from build123d import *

# Parameters (mm, degrees)
F1_DEPTH = 20
F2_R     = 10
F3_R     = 2
F4_DEPTH = 30


with BuildPart() as f1:
    # F0 (on Top) → F1 (new body)
    with BuildSketch(Plane.XY):
        with BuildLine():
            ThreePointArc((-11, 0), (0, 11), (11, 0))
            Line((11, 0), (15, 0))
            ThreePointArc((15, 0), (0, 15), (-15, 0))
            Line((-15, 0), (-11, 0))
        make_face()
        with BuildLine():
            Line((15, 0), (11, 0))
            Line((11, 0), (11, -10.1980390272))
            ThreePointArc((11, -10.1980390272), (13.9642400438, -5.4772255751), (15, 0))
        make_face()
        with BuildLine():
            Line((-11, -10.1980390272), (-11, 0))
            Line((-11, 0), (-15, 0))
            ThreePointArc((-15, 0), (-13.9642400438, -5.4772255751), (-11, -10.1980390272))
        make_face()
        with BuildLine():
            Line((11, -10.1980390272), (11, 0))
            ThreePointArc((11, 0), (0, -11), (-11, 0))
            Line((-11, 0), (-11, -10.1980390272))
            ThreePointArc((-11, -10.1980390272), (0, -15), (11, -10.1980390272))
        make_face()
        with BuildLine():
            ThreePointArc((-11, -10.1980390272), (-13.9642400438, -5.4772255751), (-15, 0))
            Line((-15, 0), (-15, -35))
            Line((-15, -35), (-11, -35))
            Line((-11, -35), (-11, -10.1980390272))
        make_face()
        with BuildLine():
            Line((15, -35), (15, 0))
            ThreePointArc((15, 0), (13.9642400438, -5.4772255751), (11, -10.1980390272))
            Line((11, -10.1980390272), (11, -35))
            Line((11, -35), (15, -35))
        make_face()
    extrude(amount=F1_DEPTH)

    # F2
    f2_edges = [f1.edges().sort_by_distance(p)[0] for p in [
        (-13, -35, 20),
        (13, -35, 20),
    ]]
    fillet(f2_edges, radius=F2_R)

    # F3 (on face) → F4 (cut)
    with BuildSketch(Plane.YZ.offset(15)):
        with Locations((-25, 10)):
            Circle(F3_R)
        with BuildLine():
            ThreePointArc((0, 8), (1.4142135624, 8.5857864376), (2, 10))
            ThreePointArc((2, 10), (1.4142135624, 11.4142135624), (0, 12))
            Line((0, 12), (0, 8))
        make_face()
        with BuildLine():
            Line((0, 8), (0, 12))
            ThreePointArc((0, 12), (-2, 10), (0, 8))
        make_face()
    extrude(amount=-F4_DEPTH, mode=Mode.SUBTRACT)


solid = f1.part
Verification items for the finished model (mm, model axes). A direction names the side the tool comes from. Coordinates: 2 decimals unless noted, no trailing zeros. Write each loop counter-clockwise with the first axis right and the second up, starting at its lowest first coordinate (ties: lowest second). Pieces come first, ordered by that corner, then holes. Notation, with made-up numbers: M 78.5,-17 L 127.5,-17 A12 ccw 127.5,1 Z; hole C 12,44.25 d11. An arc over 180 degrees is marked long. Use a Markdown table: item, result.
Q1. Sectioned sample at B-B, the plane y = -21.5. Record the boundary of the cut face in (x, z).
Reply:
| item | result |
|---|---|
| outline | M -15,0 L -11,0 L -11,20 L -15,20 Z; M 11,0 L 15,0 L 15,20 L 11,20 Z |
Q2. Set-up check for faces 4 (the face through (-11, -22.8, 9.9)), 5 (the face through (10.161, 4.213, 9.86)): record each of +Z, -Z, +X, -X, +Y, -Y from which the full face is reachable in a straight line by a thin tool's end or side.
Reply:
| item | result |
|---|---|
| face 4 | +Z, -Z, -Y |
| face 5 | +Z, -Z |
Q3. Sectioned sample at D-D, the plane y = -1.5. Record the boundary of the cut face in (x, z), plus the area to 3 significant figures.
Reply:
| item | result |
|---|---|
| outline | M -15,0 L -10.9,0 L -10.9,8.68 L -15,8.68 Z; M -15,11.32 L -10.9,11.32 L -10.9,20 L -15,20 Z; M 10.9,0 L 15,0 L 15,8.68 L 10.9,8.68 Z; M 10.9,11.32 L 15,11.32 L 15,20 L 10.9,20 Z |
| area | 142 mm² |
Q4. Sectioned sample at C-C, the plane x = -7. Record the boundary of the cut face in (y, z).
Reply:
| item | result |
|---|---|
| outline | M -13.27,0 L -8.49,0 L -8.49,20 L -13.27,20 Z; M 8.49,0 L 13.27,0 L 13.27,20 L 8.49,20 Z |
Q5. Go/stop test with flat-tipped pins: P1, Ø1, axis at x = 7, z = 5, coming from the +Y side; P2, Ø8, axis at x = -5, z = 15, coming from the -Y side; P3, Ø10, axis at x = 12, z = 17.5, coming from the -Y side; P4, Ø12, axis at x = 0.5, y = -11, coming from the -Z side. Record where each tip stops, or that it passes through.
Reply:
| item | result |
|---|---|
| P1 | stops at y = 13.52 |
| P2 | stops at y = -14.97 |
| P3 | stops at y = -34.68 |
| P4 | stops at z = 0 |
Q6. Thickness scan on line 1 (X direction, y = -21, z = 8.5); line 2 (Z direction, x = -12.25, y = -25). Record the ranges inside material, lowest first.
Reply:
| item | result |
|---|---|
| line 1 | x = -15 to -11, 11 to 15 |
| line 2 | z = 0 to 8, 12 to 20 |
Q7. Sectioned sample at A-A, the plane z = 16. Record the boundary of the cut face in (x, y).
Reply:
| item | result |
|---|---|
| outline | M -15,-33 L -11,-33 L -11,-10.2 A15 ccw 11,-10.2 L 11,-33 L 15,-33 L 15,0 A15 ccw -15,0 Z; hole C 0,0 d22 |
Q8. Draft check along Y on faces 1 (the face through (-13, -35, 5)), 2 (the face through (11, -22, 10)), 3 (the face through (-12.972, -26.474, 11.352)). Enter one of: +Y half, -Y half, draft (parallel to the pull), parting line (faces both ways), or undercut.
Reply:
| item | result |
|---|---|
| face 1 | -Y half |
| face 2 | draft |
| face 3 | undercut |
